Here's how the part is built. I have some questions about the finished solid (model axes, mm). A direction names the side the tool comes from. Give positions to 0.01 mm unless a question says otherwise; leave off trailing zeros. Order: outer loops, then holes, each group sorted by start corner. A loop starts at its lowest first (then second) coordinate and runs counter-clockwise, first axis right, second up. Notation, with made-up numbers: (29, 60) - (86, 60) arc R17 cw to (86, 72) - close; hole circle Ø4 at (2, 17.5). An arc over 180 degrees is marked (long way). One line per question, with ' | ' between items.
from build123d import *

# Parameters (mm, degrees)
BOSS_EXTRUDE1_DEPTH = 4.7
SKETCH2_R           = 1
CUT_EXTRUDE1_DEPTH  = 4.7
SKETCH3_R           = 1
CUT_EXTRUDE2_DEPTH  = 4.7


with BuildPart() as part:
    # Sketch1 → Boss-Extrude1 (new body)
    with BuildSketch(Plane(origin=(0, 0, 0), x_dir=(0, 0, -1), z_dir=(1, 0, 0))):
        Polygon((-2.453503476, 27.7), (-2.453503476, 15.9), (0.046496524, 15.9), (0, 0), (-11.8, 0), (-11.8, 1.939542533), (-2.453503476, 1.939542533), (-4.709766252, 13.909076926), (-4.709766252, 27.7), align=None)
    extrude(amount=BOSS_EXTRUDE1_DEPTH)

    # Sketch2 → Cut-Extrude1 (cut)
    with BuildSketch(Plane(origin=(0, 0, 2.453503476), x_dir=(-1, 0, 0), z_dir=(0, 0, -1))):
        with Locations(Location((-2.3, 21.8, 0), (0, 0, 90))):
            Circle(SKETCH2_R)
    extrude(amount=-CUT_EXTRUDE1_DEPTH, mode=Mode.SUBTRACT)

    # Sketch3 → Cut-Extrude2 (cut)
    with BuildSketch(Plane.XZ):
        with Locations(Location((2.3, 6.031025585, 0), (0, 0, 270))):
            Circle(SKETCH3_R)
    extrude(amount=-CUT_EXTRUDE2_DEPTH, mode=Mode.SUBTRACT)


solid = part.part
1) I want a section at D-D (x = 0.45). List the corners of the cut face in (y, z) for me, plus the area to 3 significant figures.
Model answer:
outline: (0, 0) - (15.9, -0.05) - (15.9, 2.45) - (27.7, 2.45) - (27.7, 4.71) - (13.91, 4.71) - (1.94, 2.45) - (1.94, 11.8) - (0, 11.8) - close | area: 102 mm2
2) Thinking about a two-plate mould opening in Y: for faces 6 (the face through (2, 27.7, 4)), 7 (the face through (1.692, 0.956, 6.825)), 8 (the face through (1.917, 22.724, 3.566)), which applies, +Y half, -Y half, draft (parallel to the pull), parting line (faces both ways), or undercut?
Model answer:
face 6: +Y half | face 7: draft | face 8: undercut
3) Please list where these lines run through material, in increasing order: L1, parallel to X at y = 21.8, z = 3.95; L2, parallel to Y at x = 0.5, z = 10.75; L3, parallel to Z at x = 3.4, y = 20.25.
Model answer:
L1: x = 0 to 1.3, 3.3 to 4.7 | L2: y = 0 to 1.94 | L3: z = 2.45 to 4.71
4) I'm going to push flat-ended pins straight in: P1, Ø1.4, axis at x = 1.5, y = 23, coming from the -Z side; P2, Ø1.8, axis at x = 2.3, y = 21.8, coming from the -Z side; P3, Ø1, axis at x = 0.5, z = 9.5, coming from the +Y side; P4, Ø2, axis at x = 2, y = 7, coming from the +Z side. Where does each tip first touch, or does it pass through?
Model answer:
P1: stops at z = 2.45 | P2: passes through | P3: stops at y = 1.94 | P4: stops at z = 3.6
5) I want a section at C-C (z = 5.75). List the corners of the cut face in (x, y) for me.
Model answer:
outline: (0, 0) - (1.34, 0) - (1.34, 1.94) - (0, 1.94) - close; (3.26, 0) - (4.7, 0) - (4.7, 1.94) - (3.26, 1.94) - close
6) I want a section at B-B (y = 21.8). List the corners of the cut face in (x, z) for me, plus the area to 3 significant figures.
Model answer:
outline: (0, 2.45) - (1.3, 2.45) - (1.3, 4.71) - (0, 4.71) - close; (3.3, 2.45) - (4.7, 2.45) - (4.7, 4.71) - (3.3, 4.71) - close | area: 6.09 mm2
7) I want a section at A-A (x = 2.3). List the corners of the cut face in (y, z) for me, plus the area to 3 significant figures.
Model answer:
outline: (0, 0) - (15.9, -0.05) - (15.9, 2.45) - (20.8, 2.45) - (20.8, 4.71) - (13.91, 4.71) - (1.94, 2.45) - (1.94, 5.03) - (0, 5.03) - close; (0, 7.03) - (1.94, 7.03) - (1.94, 11.8) - (0, 11.8) - close; (22.8, 2.45) - (27.7, 2.45) - (27.7, 4.71) - (22.8, 4.71) - close | area: 93.7 mm2
8) On a 3-axis mill with a long thin cutter (end or side, diameter ignored), from which of +Z, -Z, +X, -X, +Y, -Y can I reach the whole of each face in a straight line? I mean faces 1 (the face through (0, 9.8, 3.7)), 2 (the face through (2, 15.9, 1)), 3 (the face through (2, 1, 11.8)), 4 (the face through (2.3, 1.94, 7.2)), 5 (the face through (2.8, 20.7, 4.71)). Say none if no direction works.
Model answer:
face 1: +Z, -Z, -X, +Y, -Y | face 2: -Z, +X, -X, +Y | face 3: +Z, +X, -X, +Y, -Y | face 4: +Z, +X, -X | face 5: +Z, +X, -X, +Y
